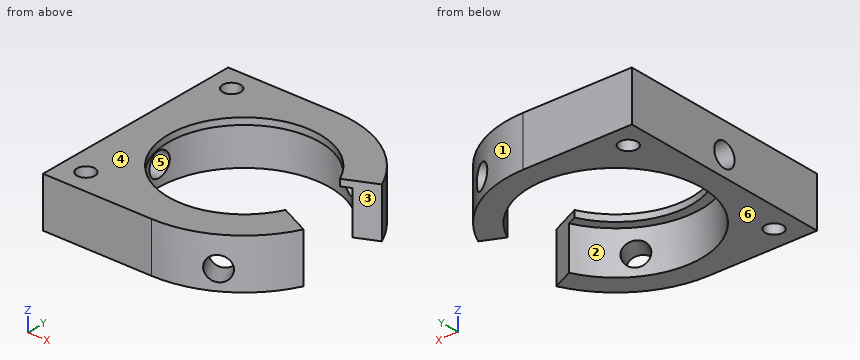
```python
from build123d import *

# Parameters (mm, degrees)
F1_DEPTH  = 7.5
F2_R      = 12.9
F3_DEPTH  = 6.5
F7_R      = 1.8
F8_DEPTH  = 10
F9_R      = 1.8
F10_DEPTH = 10
F11_R     = 1.8
F12_DEPTH = 10
F13_R     = 1.35
F14_DEPTH = 7.501


with BuildPart() as f1:
    # F0 (on Top) → F1 (new body)
    with BuildSketch(Plane.XY):
        with BuildLine():
            ThreePointArc((10.331909, -4.817848), (-11.4, 0), (10.331909, 4.817848))
            Line((10.331909, 4.817848), (14.863448, 6.930939))
            ThreePointArc((14.863448, 6.930939), (8.811714, 13.83162), (0, 16.4))
            Line((0, 16.4), (-16.4, 16.4))
            Line((-16.4, 16.4), (-16.4, -16.4))
            Line((-16.4, -16.4), (0, -16.4))
            ThreePointArc((0, -16.4), (8.811714, -13.83162), (14.863448, -6.930939))
            Line((14.863448, -6.930939), (10.331909, -4.817848))
        make_face()
    extrude(amount=F1_DEPTH)

    # F2 (on face) → F3 (cut)
    with BuildSketch(Plane(origin=(0, 0, 0), x_dir=(1, 0, 0), z_dir=(0, 0, -1))):
        Circle(F2_R)
    extrude(amount=-F3_DEPTH, mode=Mode.SUBTRACT)

    # F7 (on face) → F8 (cut)
    with BuildSketch(Plane(origin=(8.2, 14.202817, 0), x_dir=(-0.866025, 0.5, 0), z_dir=(0.5, 0.866025, 0))):
        with Locations((0, 3)):
            Circle(F7_R)
    extrude(amount=-F8_DEPTH, mode=Mode.SUBTRACT)

    # F9 (on face) → F10 (cut)
    with BuildSketch(Plane(origin=(-16.4, 0, 0), x_dir=(0, -1, 0), z_dir=(-1, 0, 0))):
        with Locations((0, 3)):
            Circle(F9_R)
    extrude(amount=-F10_DEPTH, mode=Mode.SUBTRACT)

    # F11 (on face) → F12 (cut)
    with BuildSketch(Plane(origin=(8.2, -14.202817, 0), x_dir=(0.866025, 0.5, 0), z_dir=(0.5, -0.866025, 0))):
        with Locations((0, 3)):
            Circle(F11_R)
    extrude(amount=-F12_DEPTH, mode=Mode.SUBTRACT)

    # F13 (on face) → F14 (cut, through all)
    with BuildSketch(Plane(origin=(0, 0, 0), x_dir=(1, 0, 0), z_dir=(0, 0, -1))):
        with Locations((-12.9, -12.9)):
            Circle(F13_R)
        with Locations((-12.9, 12.9)):
            Circle(F13_R)
    extrude(amount=-F14_DEPTH, mode=Mode.SUBTRACT)


solid = f1.part
```
Verification items for the finished model (mm, model axes). Face numbers are marked on the shaded views. A direction names the side the tool comes from. Round coordinates to 2 decimals unless told otherwise and drop trailing zeros. Write each loop counter-clockwise with the first axis right and the second up, starting at its lowest first coordinate (ties: lowest second). Pieces come first, ordered by that corner, then holes. Notation, with made-up numbers: (44, 70) -> (50, 70) arc R29 ccw to (50, 90) -> close; hole circle Ø8 at (26.25, 25). An arc over 180 degrees is marked (long way). Write each question's results on one line, items separated by ' | '. Start each with the question number.
1. Depth check by flat-ended pin: P1, Ø3, axis at y = 0, z = 3, coming from the -X side; P2, Ø1.5, axis at y = -2.5, z = 5.5, coming from the +X side. Enter the tip coordinate at first touch or a pass-through.
2. Material ranges on probe 1 along Y at (x, z) = (-12.9, 1.5); probe 2 along Z at (x, y) = (-15, 0); probe 3 along Y at (x, z) = (-7.5, 5.5), recorded low to high. Write a range as from..to.
3. Set-up check for the marked faces 1, 2 and 3: record each of +Z, -Z, +X, -X, +Y, -Y from which the full face is reachable in a straight line by a thin tool's end or side.
4. Draft check along Z on the marked faces 4, 5 and 6. Enter one of: +Z half, -Z half, draft (parallel to the pull), parting line (faces both ways), or undercut.
5. Cross-section at C-C (z = 5.5). Enter the section's corners in (x, y).
6. Cross-section at B-B (x = 4). Enter the section's corners in (y, z).
7. Cross-section at A-A (z = 3). Enter the section's corners in (x, y).
Solutions:
1) P1: passes through | P2: stops at x = -12.48
2) probe 1: y = -16.4..-14.25, -11.55..-0.99, 0.99..11.55, 14.25..16.4 | probe 2: z = 0..1.2, 4.8..7.5 | probe 3: y = -16.4..-10.5, 10.5..16.4
3) face 1: +Z, -Z, +X, +Y | face 2: -Z | face 3: +Z, -Z, +X
4) face 4: +Z half | face 5: undercut | face 6: -Z half
5) outline: (-16.4, -16.4) -> (0, -16.4) arc R16.4 ccw to (14.86, -6.93) -> (11.69, -5.45) arc R12.9 cw (long way) to (11.69, 5.45) -> (14.86, 6.93) arc R16.4 ccw to (0, 16.4) -> (-16.4, 16.4) -> close; hole circle Ø2.7 at (-12.9, -12.9); hole circle Ø2.7 at (-12.9, 12.9)
6) outline: (-15.9, 0) -> (-12.26, 0) -> (-12.26, 6.5) -> (-10.68, 6.5) -> (-10.68, 7.5) -> (-15.9, 7.5) -> close; (10.68, 6.5) -> (12.26, 6.5) -> (12.26, 0) -> (15.9, 0) -> (15.9, 7.5) -> (10.68, 7.5) -> close
7) outline: (-16.4, -16.4) -> (0, -16.4) arc R16.4 ccw to (6.59, -15.02) -> (4.83, -11.96) arc R12.9 cw to (-12.77, -1.8) -> (-16.4, -1.8) -> close; (-16.4, 1.8) -> (-12.77, 1.8) arc R12.9 cw to (4.83, 11.96) -> (6.59, 15.02) arc R16.4 ccw to (0, 16.4) -> (-16.4, 16.4) -> close; (7.95, -10.16) -> (9.71, -13.22) arc R16.4 ccw to (14.86, -6.93) -> (11.69, -5.45) arc R12.9 cw to start; (7.95, 10.16) arc R12.9 cw to (11.69, 5.45) -> (14.86, 6.93) arc R16.4 ccw to (9.71, 13.22) -> close; hole circle Ø2.7 at (-12.9, -12.9); hole circle Ø2.7 at (-12.9, 12.9)
